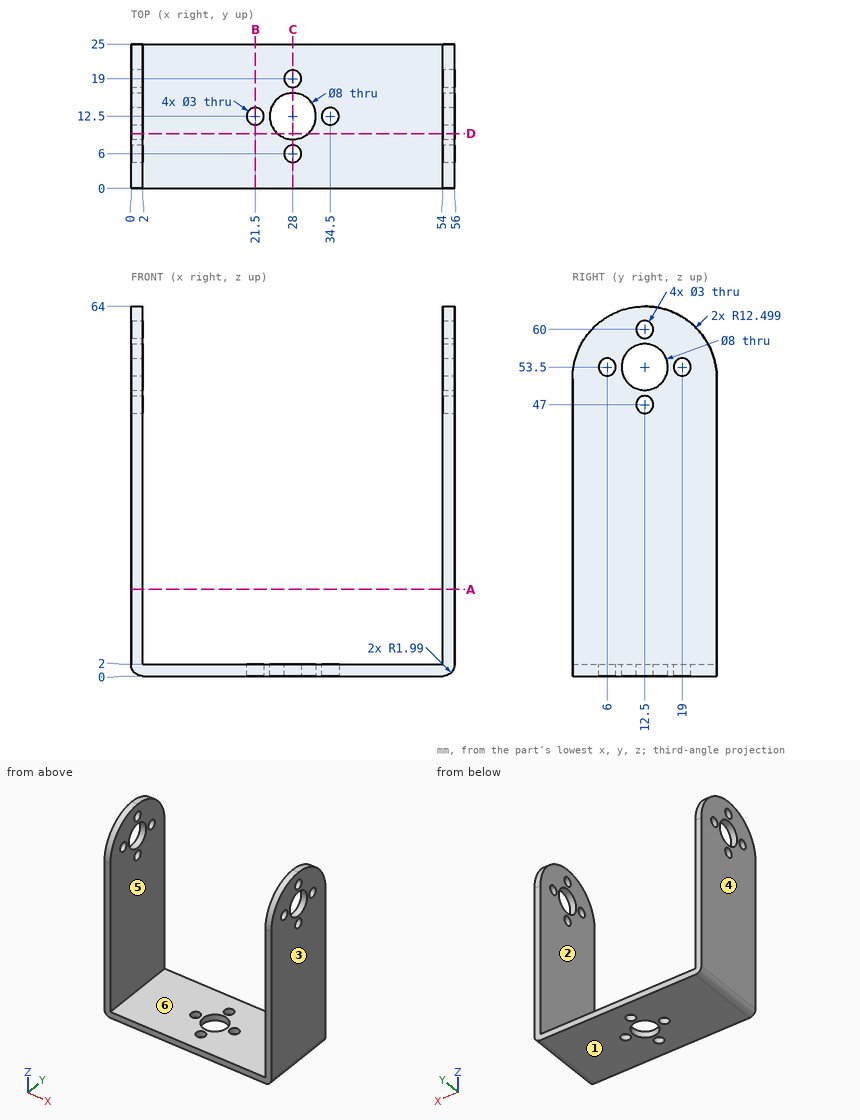
Design review of the part shown in the three views and the two pictorial views. Dimensions are in mm from the part's minimum x, y and z. A direction names the side the tool comes from. Round coordinates to 2 decimals unless told otherwise and drop trailing zeros. Order: outer loops, then holes, each group sorted by start corner. A loop starts at its lowest first (then second) coordinate and runs counter-clockwise, first axis right, second up.
Q1. We need section A-A, the plane z = 15. Give the boundary of the cut face in (x, y), plus the area to 3 significant figures.
Findings below:
outline: (0, 0) - (2, 0) - (2, 25) - (0, 25) - close; (54, 0) - (56, 0) - (56, 25) - (54, 25) - close
area: 100 mm2
Q2. We need section B-B, the plane x = 21.5. Give the boundary of the cut face in (y, z), plus the area to 3 significant figures.
Findings below:
outline: (0, 0) - (11, 0) - (11, 2) - (0, 2) - close; (14, 0) - (25, 0) - (25, 2) - (14, 2) - close
area: 44.0 mm2
Q3. We need section C-C, the plane x = 28. Give the boundary of the cut face in (y, z).
Findings below:
outline: (0, 0) - (4.5, 0) - (4.5, 2) - (0, 2) - close; (7.5, 0) - (8.5, 0) - (8.5, 2) - (7.5, 2) - close; (16.5, 0) - (17.5, 0) - (17.5, 2) - (16.5, 2) - close; (20.5, 0) - (25, 0) - (25, 2) - (20.5, 2) - close
Q4. Insertion check: P1, Ø1.8, axis at y = 12.5, z = 60, coming from the +X side; P2, Ø1.5, axis at x = 32, y = 14, coming from the +Z side. Each pin has a flat end and moves straight along its axis. Give the tip position at first contact, or say it passes through.
Findings below:
P1: passes through
P2: stops at z = 2
Q5. Wall thickness on line 1 (Y direction, x = 28, z = 1.2); line 2 (X direction, y = 23.25, z = 53); line 3 (Y direction, x = 1, z = 53): over which ranges is each line inside the solid? List them lowest first.
Findings below:
line 1: y = 0 to 4.5, 7.5 to 8.5, 16.5 to 17.5, 20.5 to 25
line 2: x = 0 to 2, 54 to 56
line 3: y = 0.09 to 4.59, 7.41 to 8.53, 16.47 to 17.59, 20.41 to 24.91
Q6. Machinability: for the marked faces 1 and 2, which of the approach directions +Z, -Z, +X, -X, +Y, -Y give a long, thin tool a straight path to every point of the face, cutting with its end or side? Answer none if there is none.
Findings below:
face 1: -Z, +X, -X, +Y, -Y
face 2: +Z, +Y, -Y
Q7. We need section D-D, the plane y = 9.5. Give the boundary of the cut face in (x, z).
Findings below:
outline: (0, 1.99) arc R1.99 ccw to (1.99, 0) - (25.35, 0) - (25.35, 2) - (2, 2) - (2, 50.85) - (0, 50.85) - close; (0, 56.15) - (2, 56.15) - (2, 63.63) - (0, 63.63) - close; (30.65, 0) - (54.01, 0) arc R1.99 ccw to (56, 1.99) - (56, 50.85) - (54, 50.85) - (54, 2) - (30.65, 2) - close; (54, 56.15) - (56, 56.15) - (56, 63.63) - (54, 63.63) - close
Q8. Mouldability with a two-part tool opening along X and no side actions: class the marked faces 3, 4, 5 and 6 as pulls with the +X half, pulls with the -X half, needs draft (parallel to the pull), parting line crosses it, or undercut.
Findings below:
face 3: pulls with the +X half
face 4: pulls with the -X half
face 5: undercut
face 6: undercut
